Geometry check sheet. Reference: the model listing, model coordinates, mm. A direction names the side the tool comes from. Coordinates: 2 decimals unless noted, no trailing zeros. Order: outer loops, then holes, each group sorted by start corner. A loop starts at its lowest first (then second) coordinate and runs counter-clockwise, first axis right, second up. Notation, with made-up numbers: M -1,-1 L 38,-1 A19 cw 38,35 Z; hole C 83.25,-8 d5. An arc over 180 degrees is marked long. One line per item, written item: value. Start each with the question number.
1) Sectioned sample at D-D, the plane x = 0. Enter the section's corners in (y, z).
2) Sectioned sample at C-C, the plane z = 5. Enter the section's corners in (x, y).
3) Sectioned sample at A-A, the plane z = 11.75. Enter the section's corners in (x, y).
4) Thickness scan on L1, parallel to Y at x = -5.75, z = 12.75; L2, parallel to X at y = 0, z = 11; L3, parallel to Y at x = 0.75, z = 11. Record the ranges inside material, lowest first. Write a range as from..to.
5) Access from +Z, -Z, +X, -X, +Y, -Y to the whole of each face (thin tool, end or side, straight path). Record for faces 4 (the flat face through (0.1, 9.5, 2)), 5 (the cylindrical face through (5.723, 1.802, 8.355)), 6 (the flat face through (-7.5, 0, 7)), 7 (the flat face through (5, 5, 13)), 8 (the cylindrical face through (0.314, -8.916, 7.395)).
6) Sectioned sample at B-B, the plane y = 7.5. Enter the section's corners in (x, z), then the cut area to 4 significant figures.
7) Draft check along Y on faces 1 (the flat face through (-6.3, -0.1, 11.3)), 2 (the flat face through (0, -10, 7)), 3 (the flat face through (0, 10, 8)). Enter one of: pulls with the +Y half, pulls with the -Y half, needs draft (parallel to the pull), parting line crosses it, or undercut.
8) Go/stop test with flat-tipped pins: P1, Ø3.5, axis at x = 6, y = -0.5, coming from the +Z side; P2, Ø0.6, axis at x = 0, z = 1, coming from the +Y side; P3, Ø0.8, axis at x = -3.5, y = 9.5, coming from the -Z side. Record where each tip stops, or that it passes through.
```python
from build123d import *

# Parameters (mm, degrees)
F0_W           = 15
F0_H           = 20
F1_DEPTH       = 15
F3_D           = 7
F3_CBORE_D     = 12
F3_CBORE_DEPTH = 11
F4_D           = 2.9
F5_W           = 10
F5_H           = 3.7
F6_DEPTH       = 15.001
F7_W           = 1
F7_H           = 2
F8_DEPTH       = 15.001


with BuildPart() as f1:
    # F0 (on Top) → F1 (new body)
    with BuildSketch(Plane.XY):
        Rectangle(F0_W, F0_H)
    extrude(amount=F1_DEPTH)

    # F3 (through all)
    with Locations(Plane.XY.offset(15)):
        with Locations((0, 0)):
            CounterBoreHole(F3_D / 2, F3_CBORE_D / 2, F3_CBORE_DEPTH)

    # F4 (through all)
    with Locations(Plane.XY.offset(15)):
        with Locations((0, -7.5), (0, 7.5)):
            Hole(F4_D / 2)

    # F5 (on face) → F6 (cut, through all)
    with BuildSketch(Plane.YZ.offset(7.5)):
        with Locations((0, 13.15)):
            Rectangle(F5_W, F5_H)
    extrude(amount=-F6_DEPTH, mode=Mode.SUBTRACT)

    # F7 (on face) → F8 (cut, through all)
    with BuildSketch(Plane.YZ.offset(7.5)):
        with Locations((9.5, 1)):
            Rectangle(F7_W, F7_H)
    extrude(amount=-F8_DEPTH, mode=Mode.SUBTRACT)


solid = f1.part
```
Final values:
1. outline: M -10,0 L -8.95,0 L -8.95,15 L -10,15 Z; M -6.05,0 L -3.5,0 L -3.5,4 L -6,4 L -6,15 L -6.05,15 Z; M 3.5,0 L 6.05,0 L 6.05,15 L 6,15 L 6,4 L 3.5,4 Z; M 8.95,0 L 9,0 L 9,2 L 10,2 L 10,15 L 8.95,15 Z
2. outline: M -7.5,-10 L 7.5,-10 L 7.5,10 L -7.5,10 Z; hole C 0,0 d12; hole C 0,-7.5 d2.9; hole C 0,7.5 d2.9
3. outline: M -7.5,-10 L 7.5,-10 L 7.5,-5 L 3.32,-5 A6 cw -3.32,-5 L -7.5,-5 Z; M -7.5,5 L -3.32,5 A6 cw 3.32,5 L 7.5,5 L 7.5,10 L -7.5,10 Z; hole C 0,-7.5 d2.9; hole C 0,7.5 d2.9
4. L1: y = -10..-5, 5..10
4. L2: x = -7.5..-6, 6..7.5
4. L3: y = -10..-8.74, -6.26..-5.95, 5.95..6.26, 8.74..10
5. face 4: -Z, +X, -X, +Y
5. face 5: +Z
5. face 6: +Z, -Z, -X, +Y, -Y
5. face 7: +Z, +X, -X
5. face 8: +Z, -Z
6. outline: M -7.5,0 L -1.45,0 L -1.45,15 L -7.5,15 Z; M 1.45,0 L 7.5,0 L 7.5,15 L 1.45,15 Z
6. area: 181.5 mm^2
7. face 1: undercut
7. face 2: pulls with the -Y half
7. face 3: pulls with the +Y half
8. P1: stops at z = 11.3
8. P2: stops at y = 9
8. P3: stops at z = 2
